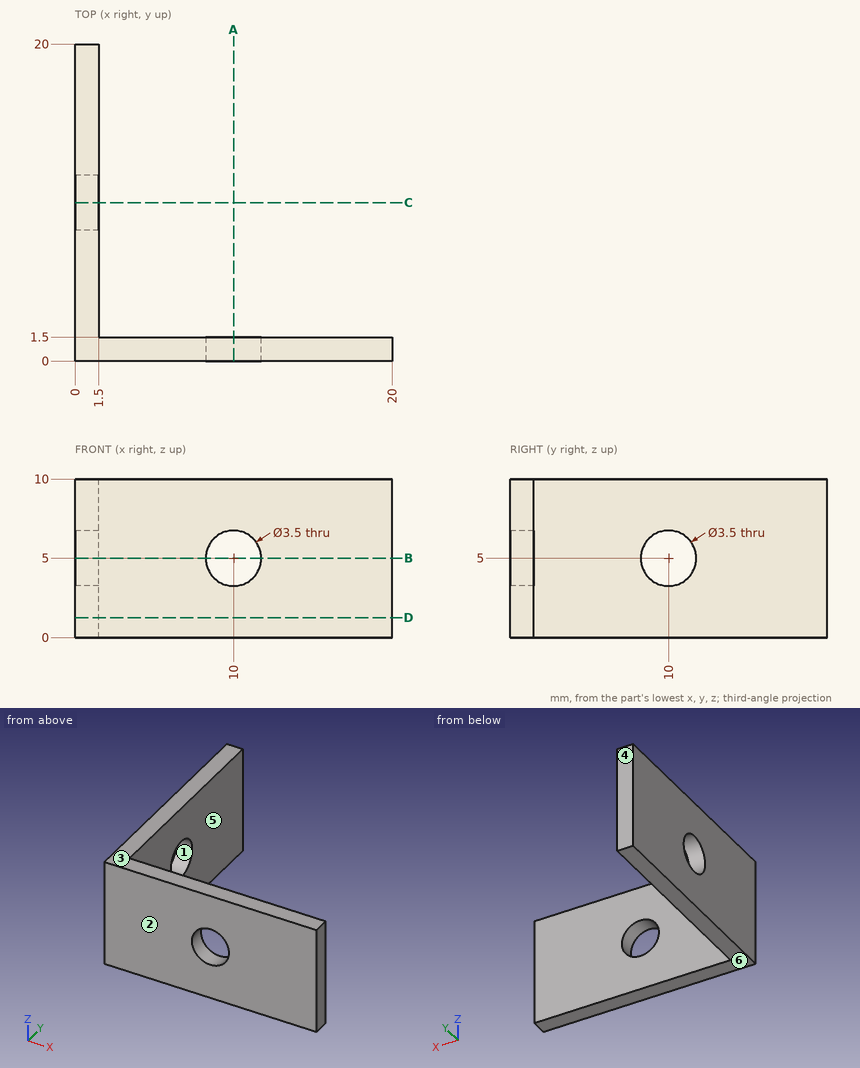
Geometry check sheet. Reference: drawing and pictorial views, mm from the part's lowest x, y, z. A direction names the side the tool comes from. Give positions to 0.01 mm unless a question says otherwise; leave off trailing zeros. Loops run counter-clockwise (first coordinate to the right, second up) from the corner with the lowest first, then second, coordinate; pieces in that order, holes last. Notation, with made-up numbers: M 23,83.25 L 72,83.25 A10 ccw 72,92.25 Z; hole C -39.75,-4.5 d11. An arc over 180 degrees is marked long. Use a Markdown table: item, result. Add a question column.
Q1. Scan lines: line 1 along Z through (x, y) = (0.65, 10); line 2 along X through (y, z) = (13.5, 2.75). Record each from-to range of solid material in increasing order. Write a range as [from, to].
Q2. Sectioned sample at B-B, the plane z = 5. Record the cut outline in (x, y), then the cut area to 4 significant figures.
Q3. Mould release check, pull along Y, two halves, no side actions. Record for the marked faces 1, 2, 3 and 4: pulls with the +Y half, pulls with the -Y half, needs draft (parallel to the pull), parting line crosses it, or undercut.
Q4. Go/stop test with flat-tipped pins: pin 1 (3 mm diameter, centred on x = 8, z = 1.5, fed in from +Y); pin 2 (3 mm diameter, centred on y = 9, z = 3, fed in from +X); pin 3 (10 mm diameter, centred on x = 8.5, y = 16.5, fed in from -Z). Record where each tip stops, or that it passes through.
Q5. Sectioned sample at A-A, the plane x = 10. Record the cut outline in (y, z).
Q6. Tool access check on the marked faces 5 and 6. Record the directions out of +Z, -Z, +X, -X, +Y, -Y that give a thin tool (end or side, any length) a straight path to the whole face; none if there is none.
Q7. Sectioned sample at D-D, the plane z = 1.25. Record the cut outline in (x, y).
Verdict:
| question | item | result |
|---|---|---|
| 1 | line 1 | [0, 3.25], [6.75, 10] |
| 1 | line 2 | [0, 1.5] |
| 2 | outline | M 0,0 L 8.25,0 L 8.25,1.5 L 1.5,1.5 L 1.5,8.25 L 0,8.25 Z; M 0,11.75 L 1.5,11.75 L 1.5,20 L 0,20 Z; M 11.75,0 L 20,0 L 20,1.5 L 11.75,1.5 Z |
| 2 | area | 47.25 mm^2 |
| 3 | face 1 | undercut |
| 3 | face 2 | pulls with the -Y half |
| 3 | face 3 | needs draft |
| 3 | face 4 | pulls with the +Y half |
| 4 | pin 1 | y = 1.5 |
| 4 | pin 2 | x = 1.5 |
| 4 | pin 3 | through |
| 5 | outline | M 0,0 L 1.5,0 L 1.5,3.25 L 0,3.25 Z; M 0,6.75 L 1.5,6.75 L 1.5,10 L 0,10 Z |
| 6 | face 5 | +Z, -Z, +X, +Y |
| 6 | face 6 | -Z, +X, -X, +Y, -Y |
| 7 | outline | M 0,0 L 20,0 L 20,1.5 L 1.5,1.5 L 1.5,20 L 0,20 Z |
